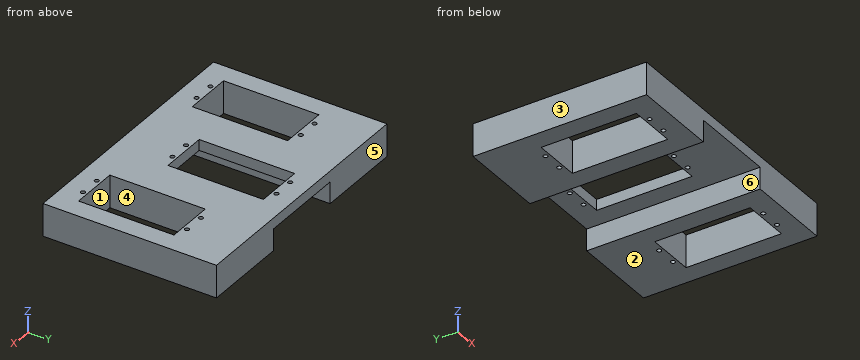
from build123d import *

# Parameters (mm, degrees)
SKETCH1_W           = 120
SKETCH1_H           = 80
BOSS_EXTRUDE1_DEPTH = 7.5
SKETCH2_R           = 1
SKETCH2_W           = 22
SKETCH2_H           = 44
CUT_EXTRUDE1_DEPTH  = 15
CUT_EXTRUDE2_REACH  = 102.281
SKETCH3_W           = 40
SKETCH3_H           = 10


with BuildPart() as part:
    # Sketch1 → Boss-Extrude1 (new, symmetric)
    with BuildSketch(Plane.XY):
        Rectangle(SKETCH1_W, SKETCH1_H)
    extrude(amount=BOSS_EXTRUDE1_DEPTH, both=True)

    # Sketch2 → Cut-Extrude1 (cut)
    with BuildSketch(Plane.XY.offset(7.5)):
        with Locations((-44.85, -31.5)):
            Circle(SKETCH2_R)
        with Locations((-35.15, -31.5)):
            Circle(SKETCH2_R)
        with Locations((-35.15, 16.5)):
            Circle(SKETCH2_R)
        with Locations((-44.85, 16.5)):
            Circle(SKETCH2_R)
        with Locations((35.15, -31.5)):
            Circle(SKETCH2_R)
        with Locations((44.85, -31.5)):
            Circle(SKETCH2_R)
        with Locations((44.85, 16.5)):
            Circle(SKETCH2_R)
        with Locations((35.15, 16.5)):
            Circle(SKETCH2_R)
        with Locations((-4.85, -16.5)):
            Circle(SKETCH2_R)
        with Locations((4.85, -16.5)):
            Circle(SKETCH2_R)
        with Locations((4.85, 31.5)):
            Circle(SKETCH2_R)
        with Locations((-4.85, 31.5)):
            Circle(SKETCH2_R)
        with Locations((-40, -7.5)):
            Rectangle(SKETCH2_W, SKETCH2_H)
        with Locations((40, -7.5)):
            Rectangle(SKETCH2_W, SKETCH2_H)
        with Locations((0, 7.5)):
            Rectangle(SKETCH2_W, SKETCH2_H)
    extrude(amount=-CUT_EXTRUDE1_DEPTH, mode=Mode.SUBTRACT)

    # Cut-Extrude2: up to this face of the body (flat: up to its plane)
    cut_extrude2_end = Plane(part.part.faces().sort_by_distance((0, -40, 0))[0])
    # Sketch3 → Cut-Extrude2 (cut, up to the picked face)
    with BuildSketch(Plane(origin=(0, 40, 0), x_dir=(1, 0, 0), z_dir=(0, 1, 0)), mode=Mode.PRIVATE) as cut_extrude2_sk1:
        with Locations((0, 2.5)):
            Rectangle(SKETCH3_W, SKETCH3_H)
    cut_extrude2_tool1 = split(extrude(cut_extrude2_sk1.sketch, amount=-CUT_EXTRUDE2_REACH, mode=Mode.PRIVATE), bisect_by=cut_extrude2_end, keep=Keep.BOTH, mode=Mode.PRIVATE)
    add(cut_extrude2_tool1.solids().sort_by(Axis((0, 40, -2.5), (0, -1, 0)))[0], mode=Mode.SUBTRACT)


solid = part.part
Design review of the part built by this model. Coordinates are the model's own, in mm. Face numbers are marked on the shaded views. A direction names the side the tool comes from. Round coordinates to 2 decimals unless told otherwise and drop trailing zeros. Write each loop counter-clockwise with the first axis right and the second up, starting at its lowest first coordinate (ties: lowest second). Pieces come first, ordered by that corner, then holes.
Item 1: Draft analysis for pull direction X (two halves, no side actions). For the marked faces 1, 2 and 3, state which applies: released by +X, released by -X, zero draft, split by the parting line, or undercut.
Item 2: For the marked faces 4, 5 and 6, list the 3-axis set-ups (+Z, -Z, +X, -X, +Y, -Y) from which the entire face can be reached by the end or side of a thin tool; tool diameter is ignored.
Item 3: Consider section D-D on y = -0.5. Give the boundary of the cut face in (x, z), and give its area (3 significant figures).
Item 4: For pin 1 Ø1.6 at (x, y) = (-4.85, -16.5) entering from +Z; pin 2 Ø4 at (x, y) = (-11.5, 0.5) entering from -Z, all flat-tipped, find the tip position at first contact; note any pin that passes through.
Item 5: Consider section A-A on z = -2. Count the separate pieces of the cut face and the enclosed holes in it, and give its area (3 significant figures).
Item 6: Consider section C-C on x = -31. Give the boundary of the cut face in (y, z), and give its area (3 significant figures).
Item 7: Wall thickness on L1, parallel to Y at x = -4.85, z = 5.25; L2, parallel to X at y = -14.5, z = 0.75; L3, parallel to Y at x = -35.15, z = 2.75: over which ranges is each line inside the solid? List them lowest first.
Check values:
1. face 1: undercut
1. face 2: zero draft
1. face 3: released by -X
2. face 4: +Z, -Z
2. face 5: +Z, -Z, +X, -X, +Y
2. face 6: -Z, +Y, -Y
3. outline: (-60, -7.5) - (-51, -7.5) - (-51, 7.5) - (-60, 7.5) - close; (-29, -7.5) - (-20, -7.5) - (-20, 2.5) - (-11, 2.5) - (-11, 7.5) - (-29, 7.5) - close; (11, 2.5) - (20, 2.5) - (20, -7.5) - (29, -7.5) - (29, 7.5) - (11, 7.5) - close; (51, -7.5) - (60, -7.5) - (60, 7.5) - (51, 7.5) - close
3. area: 630 mm2
4. pin 1: passes through
4. pin 2: stops at z = 2.5
5. separate pieces: 2
5. enclosed holes: 10
5. area: 4,440 mm2
6. outline: (-40, -7.5) - (-29.5, -7.5) - (-29.5, 7.5) - (-40, 7.5) - close; (14.5, -7.5) - (40, -7.5) - (40, 7.5) - (14.5, 7.5) - close
6. area: 540 mm2
7. L1: y = -40 to -17.5, -15.5 to -14.5, 29.5 to 30.5, 32.5 to 40
7. L2: x = -60 to -51, -29 to -20, 20 to 29, 51 to 60
7. L3: y = -40 to -32.5, -30.5 to -29.5, 14.5 to 15.5, 17.5 to 40
